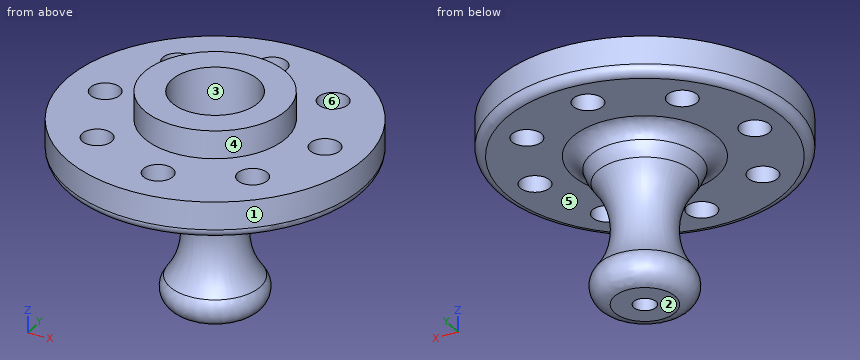
Autodesk Fusion 360 part; units mm, degrees
sketch "Sketch1" plane through (0, 0, 0) normal (0, 0, 1) x (1, 0, 0)
  circle A0 centre (0, 0) radius 0.6
  circle A1 centre (0, 0) radius 8
  circle A2 centre (0, 0) radius 2.325
  circle A3 centre (0, 0) radius 3.825
  line L0 (3.825, 0.0013) -> (5.825, 0.0013) construction
  circle A4 centre (5.825, 0.0013) radius 0.8
  circle A5 centre (4.118, 4.1198) radius 0.8
  circle A6 centre (-0.0013, 5.825) radius 0.8
  circle A7 centre (-4.1198, 4.118) radius 0.8
  circle A8 centre (-5.825, -0.0013) radius 0.8
  circle A9 centre (-4.118, -4.1198) radius 0.8
  circle A10 centre (0.0013, -5.825) radius 0.8
  circle A11 centre (4.1198, -4.118) radius 0.8
  dimension "d1" = 1.2
  dimension "d2" = 16
  dimension "d3" = 4.65
  dimension "d4" = 7.65
  dimension "d5" = 2
  dimension "d6" = 1.6
  dimension "d8" = 360
extrude "Extrude1" add sketch "Sketch1" against normal blind 2 contours A1 | A3
extrude "Extrude2" add sketch "Sketch1" along normal blind 1.5 contours A3
sketch "Sketch2" plane through (0, 0, 0) normal (1, 0, 0) x (0, 1, 0)
  line L0 (0, 0) -> (0, -10)
  line L1 (0, -10) -> (3, -10)
  line L2 (0, -2) -> (3, -2)
  line L3 (3, -10) -> (3, -9)
  line L4 (3, -2) -> (3, -3)
  arc A0 (3, -3) -> (3, -9) centre (5.5787, -6) ccw
  dimension "d13" = 10
  dimension "d14" = 3
  dimension "d24" = 1
  dimension "d25" = 1
revolve "Revolve2" add sketch "Sketch2" angle 360 about axis through (0, 0, 1.75) along (0, 0, 1)
fillet "Fillet4" radius 2 1 edges at (-2.797, 1.0848, -9)
fillet "Fillet5" radius 2 1 edges at (-2.797, 1.0848, -3)
fillet "Fillet6" radius 1 1 edges at (-2.797, 1.0848, -10)
extrude "Extrude3" cut sketch "Sketch1" against normal blind 11 contours A0
fillet "Fillet8" radius 1 1 edges at (1.0848, -2.797, -2)
fillet "Fillet9" radius 0.5 1 edges at (-7.4586, 2.8929, -2)
revolve "Revolve1" [suppressed]
fillet "Fillet1" [suppressed]
fillet "Fillet2" [suppressed]
fillet "Fillet3" [suppressed]
Geometry check sheet. Reference: the model listing, model coordinates, mm. Face numbers are marked on the shaded views. A direction names the side the tool comes from. Give positions to 0.01 mm unless a question says otherwise; leave off trailing zeros. Write each question's results on one line, items separated by ' | '.
1) Release check for a two-part mould opening along X. For the marked faces 1, 2 and 3 record: +X half, -X half, draft (parallel to the pull), parting line (faces both ways), or undercut.
Answers follow:
face 1: parting line | face 2: draft | face 3: undercut
2) Tool access check on the marked faces 4, 5 and 6. Record the directions out of +Z, -Z, +X, -X, +Y, -Y that give a thin tool (end or side, any length) a straight path to the whole face; none if there is none.
Answers follow:
face 4: +Z | face 5: -Z | face 6: +Z, -Z
3) Thickness scan on line 1 (Y direction, x = 0, z = 0.5) (3 decimals); line 2 (Z direction, x = 3, y = -4); line 3 (X direction, y = 1.5, z = -1.75). Record the ranges inside material, lowest first.
Answers follow:
line 1: -3.825 to -2.325, 2.325 to 3.825 | line 2: -2 to 0 | line 3: -7.79 to -1.78, 1.78 to 7.79
4) Gauge pin test, flat ends, axial feed: pin 1 (5.5 mm diameter, centred on x = 0, y = 0, fed in from +Z); pin 2 (1.4 mm diameter, centred on x = -1, y = 0.5, fed in from +Z); pin 3 (1.5 mm diameter, centred on y = 1, z = -4, fed in from -X); pin 4 (1.5 mm diameter, centred on x = -1, z = -5.5, fed in from +Y). Record the tip position at first contact, or that the pin passes through.
Answers follow:
pin 1: z = 1.5 | pin 2: z = -2 | pin 3: x = -2.56 | pin 4: y = 1.7
5) Section check A-A, the plane x = 0. Count the separate pieces of the cut face and the enclosed holes in it, plus the area to 3 significant figures.
Answers follow:
separate pieces: 4 | enclosed holes: 0 | area: 46.5 mm2
